Model file for the job. Use its own axes, mm. A direction names the side the tool comes from. Give positions to 0.01 mm unless a question says otherwise; leave off trailing zeros. Order: outer loops, then holes, each group sorted by start corner. A loop starts at its lowest first (then second) coordinate and runs counter-clockwise, first axis right, second up. Notation, with made-up numbers: (36, 66.5) -> (47, 66.5) arc R33 ccw to (47, 105.5) -> close; hole circle Ø7 at (-8, 83). An arc over 180 degrees is marked (long way). Answer in a Markdown table with one row per item. Add a question column.
from build123d import *

# Parameters (mm, degrees)
SKETCH_1_R      = 5
EXTRUDE_1_DEPTH = 35.15
SKETCH_2_R      = 1.5
EXTRUDE_2_DEPTH = 3.7
SKETCH_3_R      = 1.5
EXTRUDE_3_DEPTH = 3.7


with BuildPart() as part:
    # 草图1 → 凸台-拉伸1 (new body)
    with BuildSketch(Plane.XY):
        Circle(SKETCH_1_R)
    extrude(amount=EXTRUDE_1_DEPTH)

    # 草图2 → 凸台-拉伸2 (add)
    with BuildSketch(Plane(origin=(0, 0, 0), x_dir=(-1, 0, 0), z_dir=(0, 0, -1))):
        Circle(SKETCH_2_R)
    extrude(amount=EXTRUDE_2_DEPTH)

    # 草图3 → 凸台-拉伸3 (add)
    with BuildSketch(Plane.XY.offset(35.15)):
        Circle(SKETCH_3_R)
    extrude(amount=EXTRUDE_3_DEPTH)


solid = part.part
Item 1: Pin check, flat tips, straight feed: pin 1 Ø1.5 at (x, z) = (-2.5, 3.5) entering from -Y; pin 2 Ø3 at (x, z) = (-4, 13.5) entering from -Y; pin 3 Ø2 at (x, y) = (-3.5, -2) entering from +Z. Stop position of each tip, or through.
Item 2: Saw through at D-D on x = -3. List the corners of the cut face in (y, z), plus the area to 3 significant figures.
Item 3: Saw through at C-C on z = 1. List the corners of the cut face in (x, y), plus the area to 3 significant figures.
Item 4: Which spindle directions (+Z, -Z, +X, -X, +Y, -Y) get a long thin tool onto all of the face, cutting with end or side? Do faces 1 (the flat face through (-1.2, 1.2, 0)), 2 (the flat face through (-1.2, 1.2, 35.15)), 3 (the cylindrical face through (-1.08, -4.88, 17.33)). Say none if no direction does.
Item 5: Saw through at A-A on y = 0. List the corners of the cut face in (x, z).
Item 6: Wall check: line 1 (Y direction, x = -0.25, z = 14.5); line 2 (Z direction, x = 0, y = -2.5); line 3 (Y direction, x = -2.5, z = 20.5). Give the ranges that are in metal, low to high.
Evaluation:
| question | item | result |
|---|---|---|
| 1 | pin 1 | stops at y = -4.68 |
| 1 | pin 2 | stops at y = -4.33 |
| 1 | pin 3 | stops at z = 35.15 |
| 2 | outline | (-4, 0) -> (4, 0) -> (4, 35.15) -> (-4, 35.15) -> close |
| 2 | area | 281 mm2 |
| 3 | outline | circle Ø10 at (0, 0) |
| 3 | area | 78.5 mm2 |
| 4 | face 1 | -Z |
| 4 | face 2 | +Z |
| 4 | face 3 | +Z, -Z |
| 5 | outline | (-5, 0) -> (-1.5, 0) -> (-1.5, -3.7) -> (1.5, -3.7) -> (1.5, 0) -> (5, 0) -> (5, 35.15) -> (1.5, 35.15) -> (1.5, 38.85) -> (-1.5, 38.85) -> (-1.5, 35.15) -> (-5, 35.15) -> close |
| 6 | line 1 | y = -4.99 to 4.99 |
| 6 | line 2 | z = 0 to 35.15 |
| 6 | line 3 | y = -4.33 to 4.33 |
